Geometry: final body of the model. Coordinates: model frame, mm. Face numbers are marked on the shaded views. A direction names the side the tool comes from. Give positions to 0.01 mm unless a question says otherwise; leave off trailing zeros. Loops run counter-clockwise (first coordinate to the right, second up) from the corner with the lowest first, then second, coordinate; pieces in that order, holes last.
from build123d import *

# Parameters (mm, degrees)
SKETCH1_W           = 95
SKETCH1_H           = 37.8
BOSS_EXTRUDE1_DEPTH = 3.6
SKETCH2_R           = 1.4
CUT_EXTRUDE1_DEPTH  = 4
SKETCH3_W           = 6
SKETCH3_H           = 6
SKETCH3_W_2         = 7
SKETCH3_H_2         = 5
SKETCH3_W_3         = 5
CUT_EXTRUDE5_DEPTH  = 1.5
BOSS_EXTRUDE3_DEPTH = 1.5
SKETCH6_W           = 15
SKETCH6_H           = 5
CUT_EXTRUDE6_DEPTH  = 18.5
SKETCH7_W           = 10
SKETCH7_H           = 1.5
CUT_EXTRUDE7_DEPTH  = 2
SKETCH9_W           = 23
SKETCH9_H           = 1.5
CUT_EXTRUDE8_DEPTH  = 1.5
SKETCH10_W          = 18
SKETCH10_H          = 1.5
BOSS_EXTRUDE5_DEPTH = 1.5
SKETCH11_W          = 34.32
SKETCH11_H          = 28.9
SKETCH11_W_2        = 23.5
CUT_EXTRUDE10_DEPTH = 1.2
SKETCH12_W          = 1.5
SKETCH12_H          = 1.5
BOSS_EXTRUDE6_DEPTH = 0.5


with BuildPart() as part:
    # Sketch1 → Boss-Extrude1 (new body)
    with BuildSketch(Plane(origin=(0, 0, 0), x_dir=(1, 0, 0), z_dir=(0, 1, 0))):
        Rectangle(SKETCH1_W, SKETCH1_H)
    extrude(amount=BOSS_EXTRUDE1_DEPTH)

    # Sketch2 → Cut-Extrude1 (cut)
    with BuildSketch(Plane(origin=(0, 3.6, 0), x_dir=(1, 0, 0), z_dir=(0, 1, 0))):
        with Locations((-42.82, -0.18)):
            Circle(SKETCH2_R)
        with Locations((-19.96, 15.7)):
            Circle(SKETCH2_R)
        with Locations((24.5, -2.72)):
            Circle(SKETCH2_R)
    extrude(amount=-CUT_EXTRUDE1_DEPTH, mode=Mode.SUBTRACT)

    # Sketch3 → Cut-Extrude5 (cut)
    with BuildSketch(Plane.XZ):
        with Locations((-37.82, -9.62)):
            Rectangle(SKETCH3_W, SKETCH3_H)
        Polygon((28, -18.9), (7, -18.9), (7, -8.9), (11, -8.9), (28, -8.9), align=None)
        with BuildLine():
            Line((-19.26, -6.1), (-19.26, 15.9))
            Line((-19.26, 15.9), (22.74, 15.9))
            Line((22.74, 15.9), (22.74, 4.12))
            Line((22.74, 4.12), (24.5, 4.12))
            ThreePointArc((24.5, 4.12), (25.9, 2.72), (24.5, 1.32))
            Line((24.5, 1.32), (22.74, 1.32))
            Line((22.74, 1.32), (22.74, -6.1))
            Line((22.74, -6.1), (-19.26, -6.1))
        make_face()
        with Locations((42, -14.4)):
            Rectangle(SKETCH3_W_2, SKETCH3_H_2)
        with Locations((-14.76, -16.4)):
            Rectangle(SKETCH3_W_3, SKETCH3_H_2)
    extrude(amount=-CUT_EXTRUDE5_DEPTH, mode=Mode.SUBTRACT)

    # Sketch4 → Boss-Extrude3 (add)
    with BuildSketch(Plane.XZ.offset(-1.5)):
        with BuildLine():
            Line((22.74, 4.12), (22.74, 15.9))
            Line((22.74, 15.9), (20.74, 15.9))
            Line((20.74, 15.9), (20.74, 4.12))
            Line((20.74, 4.12), (20.74, -6.1))
            Line((20.74, -6.1), (22.74, -6.1))
            Line((22.74, -6.1), (22.74, 1.32))
            Line((22.74, 1.32), (24.5, 1.32))
            ThreePointArc((24.5, 1.32), (23.1, 2.72), (24.5, 4.12))
            Line((24.5, 4.12), (22.74, 4.12))
        make_face()
    extrude(amount=BOSS_EXTRUDE3_DEPTH)

    # Sketch6 → Cut-Extrude6 (cut)
    with BuildSketch(Plane(origin=(0, 3.6, 0), x_dir=(1, 0, 0), z_dir=(0, 1, 0))):
        with Locations((16, 13.4)):
            Rectangle(SKETCH6_W, SKETCH6_H)
    extrude(amount=-CUT_EXTRUDE6_DEPTH, mode=Mode.SUBTRACT)

    # Sketch7 → Cut-Extrude7 (cut)
    with BuildSketch(Plane.ZY.offset(-28)):
        with Locations((-13.9, 0.75)):
            Rectangle(SKETCH7_W, SKETCH7_H)
    extrude(amount=-CUT_EXTRUDE7_DEPTH, mode=Mode.SUBTRACT)

    # Sketch9 → Cut-Extrude8 (cut)
    with BuildSketch(Plane(origin=(0, 0, -8.9), x_dir=(-1, 0, 0), z_dir=(0, 0, -1))):
        with Locations((-18.5, 0.75)):
            Rectangle(SKETCH9_W, SKETCH9_H)
    extrude(amount=-CUT_EXTRUDE8_DEPTH, mode=Mode.SUBTRACT)

    # Sketch10 → Boss-Extrude5 (add)
    with BuildSketch(Plane.XZ.offset(-1.5)):
        with Locations((21, -18.15)):
            Rectangle(SKETCH10_W, SKETCH10_H)
    extrude(amount=BOSS_EXTRUDE5_DEPTH)

    # Sketch11 → Cut-Extrude10 (cut)
    with BuildSketch(Plane(origin=(0, 3.6, 0), x_dir=(1, 0, 0), z_dir=(0, 1, 0))):
        with Locations((-22.66, -4.45)):
            Rectangle(SKETCH11_W, SKETCH11_H)
        with Locations((10.25, -4.45)):
            Rectangle(SKETCH11_W_2, SKETCH11_H)
    extrude(amount=-CUT_EXTRUDE10_DEPTH, mode=Mode.SUBTRACT)

    # Sketch12 → Boss-Extrude6 (add)
    with BuildSketch(Plane.ZY.offset(-12)):
        with Locations((-18.15, 0.75)):
            Rectangle(SKETCH12_W, SKETCH12_H)
    extrude(amount=BOSS_EXTRUDE6_DEPTH)


solid = part.part
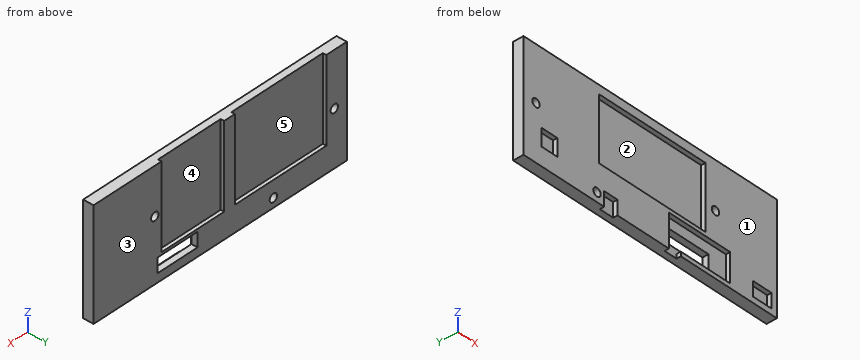
Item 1: Section query B-B on z = 2.72. Return loops of the section in (x, y), plus the area to 3 significant figures.
Values follow:
outline: (-47.5, 0) - (-19.26, 0) - (-19.26, 1.5) - (20.74, 1.5) - (20.74, 0) - (23.1, 0) - (23.1, 3.6) - (22, 3.6) - (22, 2.4) - (-1.5, 2.4) - (-1.5, 3.6) - (-5.5, 3.6) - (-5.5, 2.4) - (-39.82, 2.4) - (-39.82, 3.6) - (-47.5, 3.6) - close; (25.9, 0) - (47.5, 0) - (47.5, 3.6) - (25.9, 3.6) - close
area: 203 mm2
Item 2: Draft query along X for the marked faces 3, 4 and 5. Return one class per face: +X half, -X half, draft (parallel to the pull), parting line (faces both ways), or undercut.
Values follow:
face 3: draft
face 4: undercut
face 5: undercut
Item 3: Set-up query: the marked faces 1 and 2. Return all of +Z, -Z, +X, -X, +Y, -Y with unobstructed straight access to the full face (end or side cutting, diameter ignored); none if empty.
Values follow:
face 1: +Z, -Z, +X, -X, -Y
face 2: -Y
Item 4: Section query A-A on x = -42.82. Return loops of the section in (y, z).
Values follow:
outline: (0, -18.9) - (3.6, -18.9) - (3.6, -1.22) - (0, -1.22) - close; (0, 1.58) - (3.6, 1.58) - (3.6, 18.9) - (0, 18.9) - close
Item 5: Ray query, probe 1 along Z at (x, y) = (24.5, 1); probe 2 along X at (y, z) = (1.6, -15.7); probe 3 along X at (y, z) = (2.7, 7.5). Return the intervals inside material, ascending.
Values follow:
probe 1: z = -18.9 to -17.4, -7.4 to 1.32, 4.12 to 18.9
probe 2: x = -47.5 to -21.36, -18.56 to 8.5, 23.5 to 47.5
probe 3: x = -47.5 to -39.82, -5.5 to -1.5, 22 to 47.5
Item 6: Section query D-D on z = 8. Return loops of the section in (x, y).
Values follow:
outline: (-47.5, 0) - (-19.26, 0) - (-19.26, 1.5) - (20.74, 1.5) - (20.74, 0) - (47.5, 0) - (47.5, 3.6) - (22, 3.6) - (22, 2.4) - (-1.5, 2.4) - (-1.5, 3.6) - (-5.5, 3.6) - (-5.5, 2.4) - (-39.82, 2.4) - (-39.82, 3.6) - (-47.5, 3.6) - close
Item 7: Pin query (flat end, axial travel): pin 1 (6 mm diameter, centred on x = 11, z = 11.5, fed in from -Y); pin 2 (2 mm diameter, centred on x = -22.5, z = 4.5, fed in from -Y); pin 3 (2.5 mm diameter, centred on x = -42.82, z = 0.18, fed in from -Y). Return the tip coordinate at first contact, or that it passes through.
Values follow:
pin 1: stops at y = 1.5
pin 2: stops at y = 0
pin 3: passes through
Item 8: Section query C-C on y = 0.85. Give the number of separate pieces and of enclosed holes in the cut face, plus the area to 3 significant figures.
Values follow:
separate pieces: 1
enclosed holes: 6
area: 2,360 mm2
